```python
from build123d import *

# Parameters (mm, degrees)
SKETCH1_W           = 79.5
SKETCH1_H           = 43
BOSS_EXTRUDE1_DEPTH = 2
SKETCH2_W           = 71.7
SKETCH2_H           = 38.8
BOSS_EXTRUDE2_DEPTH = 22.6
SKETCH3_W           = 69.7
SKETCH3_H           = 36.8
CUT_EXTRUDE1_DEPTH  = 8.5
BOSS_EXTRUDE3_DEPTH = 22.6
SKETCH6_W           = 67.219676188
SKETCH6_H           = 8.940869551
CUT_EXTRUDE2_DEPTH  = 22.6
SKETCH7_R           = 6.66374012
SKETCH7_R_2         = 5.829163104
BOSS_EXTRUDE4_DEPTH = 20.1
FILLET1_R           = 3
SKETCH8_W           = 27.801535977
SKETCH8_H           = 10.55826339
BOSS_EXTRUDE5_DEPTH = 17
SKETCH9_W           = 67.5
SKETCH9_H           = 31
CUT_EXTRUDE3_DEPTH  = 1
SKETCH10_W          = 28.845725121
SKETCH10_H          = 25.974204973
CUT_EXTRUDE4_DEPTH  = 1
SKETCH11_R          = 6.25
BOSS_EXTRUDE6_DEPTH = 12
BOSS_EXTRUDE7_START = 2.5
BOSS_EXTRUDE7_DEPTH = 11.5


with BuildPart() as part:
    # Sketch1 → Boss-Extrude1 (new body)
    with BuildSketch(Plane(origin=(0, 0, 0), x_dir=(1, 0, 0), z_dir=(0, 1, 0))):
        with Locations((25.074854651, -17.802325581)):
            Rectangle(SKETCH1_W, SKETCH1_H)
    extrude(amount=BOSS_EXTRUDE1_DEPTH)

    # Sketch2 → Boss-Extrude2 (add)
    with BuildSketch(Plane(origin=(0, 2, 0), x_dir=(1, 0, 0), z_dir=(0, 1, 0))):
        with Locations((25.074854651, -17.802325581)):
            Rectangle(SKETCH2_W, SKETCH2_H)
    extrude(amount=BOSS_EXTRUDE2_DEPTH)

    # Sketch3 → Cut-Extrude1 (cut)
    with BuildSketch(Plane(origin=(0, 24.6, 0), x_dir=(1, 0, 0), z_dir=(0, 1, 0))):
        with Locations((25.074854651, -17.802325581)):
            Rectangle(SKETCH3_W, SKETCH3_H)
    extrude(amount=-CUT_EXTRUDE1_DEPTH, mode=Mode.SUBTRACT)

    # Sketch5 → Boss-Extrude3 (add)
    with BuildSketch(Plane(origin=(0, 16.1, 0), x_dir=(1, 0, 0), z_dir=(0, 1, 0))):
        Polygon((41.224854651, -26.202325581), (-4.775145349, -26.202325581), (-4.775145349, -36.202325581), (-2.433003128, -36.202325581), (-2.433003128, -28.831573422), (3.571084453, -28.831573422), (3.571084453, -36.202325581), (5.724724564, -36.202325581), (5.724724564, -28.831573422), (12.250906718, -28.831573422), (12.250906718, -36.202325581), (14.208761365, -36.202325581), (14.208761365, -28.831573422), (20.604419876, -28.831573422), (20.604419876, -36.202325581), (22.823321808, -36.202325581), (22.823321808, -28.831573422), (28.240052996, -28.831573422), (28.240052996, -36.202325581), (30.589478571, -36.202325581), (30.589478571, -28.831573422), (38.486158978, -28.831573422), (38.486158978, -36.202325581), (41.224854651, -36.202325581), align=None)
    extrude(amount=BOSS_EXTRUDE3_DEPTH)

    # Sketch6 → Cut-Extrude2 (cut)
    with BuildSketch(Plane.XY.offset(37.202325581)):
        with Locations((18.972874337, 40.670434775)):
            Rectangle(SKETCH6_W, SKETCH6_H)
    extrude(amount=-CUT_EXTRUDE2_DEPTH, mode=Mode.SUBTRACT)

    # Sketch7 → Boss-Extrude4 (add)
    with BuildSketch(Plane(origin=(0, 16.1, 0), x_dir=(1, 0, 0), z_dir=(0, 1, 0))):
        with Locations((51.669046929, -11.341405249)):
            Circle(SKETCH7_R)
        with Locations((52.386926966, -26.090576917)):
            Circle(SKETCH7_R_2)
    extrude(amount=BOSS_EXTRUDE4_DEPTH)

    # Fillet1
    fillet1_edges = [part.edges().sort_by_distance(p)[0] for p in [
        (-14.675145349, 1, -3.697674419),
        (64.824854651, 1, -3.697674419),
        (64.824854651, 1, 39.302325581),
        (-14.675145349, 1, 39.302325581),
    ]]
    fillet(fillet1_edges, radius=FILLET1_R)

    # Sketch8 → Boss-Extrude5 (add)
    with BuildSketch(Plane(origin=(0, 16.1, 0), x_dir=(1, 0, 0), z_dir=(0, 1, 0))):
        with Locations((25.172747384, -5.279131695)):
            Rectangle(SKETCH8_W, SKETCH8_H)
    extrude(amount=BOSS_EXTRUDE5_DEPTH)

    # Sketch9 → Cut-Extrude3 (cut)
    with BuildSketch(Plane.XZ):
        with Locations((25.074854651, 17.802325581)):
            Rectangle(SKETCH9_W, SKETCH9_H)
    extrude(amount=-CUT_EXTRUDE3_DEPTH, mode=Mode.SUBTRACT)

    # Sketch10 → Cut-Extrude4 (cut)
    with BuildSketch(Plane.XZ.offset(-1)):
        with Locations((18.581303408, 17.606540116)):
            Rectangle(SKETCH10_W, SKETCH10_H)
    extrude(amount=-CUT_EXTRUDE4_DEPTH, mode=Mode.SUBTRACT)

    # Sketch11 → Boss-Extrude6 (add)
    with BuildSketch(Plane.XZ.offset(-1)):
        with Locations((50.42907232, 22.696962197)):
            Circle(SKETCH11_R)
    extrude(amount=BOSS_EXTRUDE6_DEPTH)

    # Sketch12 → Boss-Extrude7 (add)
    with BuildSketch(Plane(origin=(-9.775145349, 0, 0), x_dir=(0, 0, -1), z_dir=(1, 0, 0)).offset(BOSS_EXTRUDE7_START)):
        with BuildLine():
            Line((-23.402325581, 16.1), (-23.402325581, 27))
            ThreePointArc((-23.402325581, 27), (-12.902325581, 37.5), (-2.402325581, 27))
            Line((-2.402325581, 27), (-2.402325581, 16.1))
            ThreePointArc((-2.402325581, 16.1), (-12.902325581, 5.6), (-23.402325581, 16.1))
        make_face()
    extrude(amount=BOSS_EXTRUDE7_DEPTH)


solid = part.part
```
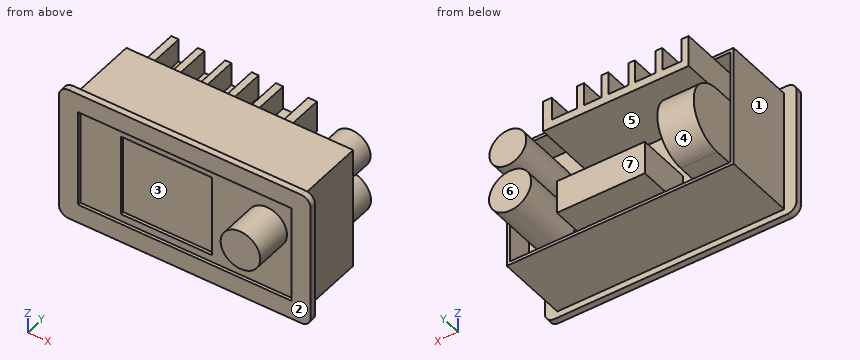
Check sheet for the modelled part. Datum: model origin and axes. Units: mm. Face numbers are marked on the shaded views. A direction names the side the tool comes from. Round coordinates to 2 decimals unless told otherwise and drop trailing zeros. Order: outer loops, then holes, each group sorted by start corner. A loop starts at its lowest first (then second) coordinate and runs counter-clockwise, first axis right, second up.
1) Section check A-A (x = 32). Record the boundary of the cut face in (y, z).
2) Mould release check, pull along X, two halves, no side actions. Record for the marked faces 1, 2 and 3: +X half, -X half, draft (parallel to the pull), parting line (faces both ways), or undercut.
3) Go/stop test with flat-tipped pins: pin 1 Ø6 at (x, z) = (36, 31.5) entering from +Y; pin 2 Ø12 at (x, z) = (7.5, 8) entering from -Y; pin 3 Ø3.5 at (y, z) = (25.5, 31) entering from +X. Record where each tip stops, or that it passes through.
4) Scan lines: line 1 (Z direction, x = 12.5, y = 20.5); line 2 (Z direction, x = 19, y = 17.5); line 3 (X direction, y = 25, z = 10). Record each from-to range of solid material in increasing order.
5) Tool access check on the marked faces 4, 5, 6 and 7. Record the directions out of +Z, -Z, +X, -X, +Y, -Y that give a thin tool (end or side, any length) a straight path to the whole face; none if there is none.
6) Section check D-D (z = 14.5). Record the boundary of the cut face in (x, y).
7) Section check B-B (y = 32). Give the number of separate pieces and of enclosed holes in the cut face, and give its area (3 significant figures).
Result:
1. outline: (0, -3.7) - (2, -3.7) - (2, -1.6) - (24.6, -1.6) - (24.6, -0.6) - (16.1, -0.6) - (16.1, 0) - (33.1, 0) - (33.1, 10.56) - (16.1, 10.56) - (16.1, 26.2) - (36.2, 26.2) - (36.2, 28.83) - (16.1, 28.83) - (16.1, 36.2) - (24.6, 36.2) - (24.6, 37.2) - (2, 37.2) - (2, 39.3) - (0, 39.3) - (0, 33.3) - (1, 33.3) - (1, 30.59) - (2, 30.59) - (2, 4.62) - (1, 4.62) - (1, 2.3) - (0, 2.3) - close
2. face 1: -X half
2. face 2: draft
2. face 3: undercut
3. pin 1: stops at y = 36.2
3. pin 2: stops at y = 0
3. pin 3: stops at x = 60.92
4. line 1: z = -1.6 to -0.6, 0 to 10.56, 26.2 to 37.2
4. line 2: z = -1.6 to -0.6, 0 to 10.56, 26.2 to 28.83, 36.2 to 37.2
4. line 3: x = -7.28 to 4.22, 11.27 to 39.07, 45.14 to 58.2
5. face 4: -X, +Y
5. face 5: +Y
5. face 6: +Z, -Z, +X, +Y
5. face 7: -Z, +Y
6. outline: (-14.68, 0) - (-8.68, 0) - (-8.68, 1) - (4.16, 1) - (4.16, 2) - (33, 2) - (33, 1) - (58.82, 1) - (58.82, 0) - (64.82, 0) - (64.82, 2) - (60.92, 2) - (60.92, 24.6) - (59.92, 24.6) - (59.92, 16.1) - (57.54, 16.1) - (57.54, 36.2) - (45.8, 36.2) - (45.8, 16.1) - (4.22, 16.1) - (4.22, 37.38) - (-7.28, 37.38) - (-7.28, 16.1) - (-9.78, 16.1) - (-9.78, 24.6) - (-10.78, 24.6) - (-10.78, 2) - (-14.68, 2) - close
7. separate pieces: 5
7. enclosed holes: 0
7. area: 975 mm2
